Design review of the part built by this model. Coordinates are the model's own, in mm. A direction names the side the tool comes from. Give positions to 0.01 mm unless a question says otherwise; leave off trailing zeros. Write each loop counter-clockwise with the first axis right and the second up, starting at its lowest first coordinate (ties: lowest second). Pieces come first, ordered by that corner, then holes. Notation, with made-up numbers: M -25,84 L -8,84 A34 ccw -8,120 Z; hole C 68.25,17 d5. An arc over 180 degrees is marked long. Answer in a Markdown table with one row per item.
```python
from build123d import *

# Parameters (mm, degrees)
F1_DEPTH = 10
F2_R     = 5
F3_R     = 2.5
F5_R     = 1.5
F6_DEPTH = 25


# Not quite as in the source:
# - two fillets or chamfers of one size are made in one step
# - a feature names something its author has since deleted; it is built from what else it names


with BuildPart() as f1:
    # F0 (on Front) → F1 (new body)
    with BuildSketch(Plane.XZ):
        Polygon((-40.5, 0), (0, 0), (0, -6.2), (7, -6.2), (7, 7.8), (-47.5, 7.8), (-47.5, -6.2), (-87.5, -46.2), (-107.5, -46.2), (-107.5, -56.2), (-87.6005050634, -56.2), (-43.6005050634, -12.2), (-34.5, -12.2), (-34.5, -6.2), (-40.5, -6.2), align=None)
    extrude(amount=F1_DEPTH)

    # F2
    f2_edges = [f1.edges().sort_by_distance(p)[0] for p in [
        (7, -5, -6.2),
        (7, -5, 7.8),
        (-47.5, -5, 7.8),
        (-47.5, -5, -6.2),
        (-87.5, -5, -46.2),
        (-87.600505, -5, -56.2),
        (-43.600505, -5, -12.2),
    ]]
    fillet(f2_edges, radius=F2_R)

    # F3
    f3_edges = [f1.edges().sort_by_distance(p)[0] for p in [
        (-34.5, -5, -12.2),
        (-34.5, -5, -6.2),
    ]]
    fillet(f3_edges, radius=F3_R)

    # F5 (on face) → F6 (cut)
    with BuildSketch(Plane(origin=(0, 0, -56.2), x_dir=(1, 0, 0), z_dir=(0, 0, -1))):
        with Locations((-102.5, 5)):
            Circle(F5_R)
        with Locations((-92.5, 5)):
            Circle(F5_R)
    extrude(amount=-F6_DEPTH, mode=Mode.SUBTRACT)


solid = f1.part
```
1) To check wall thickness, follow probe 1 along Y at (x, z) = (-92.5, -52.5); probe 2 along X at (y, z) = (-0.75, -1); probe 3 along Z at (x, y) = (-1, -8.5). State the ranges of each line that lie inside material, in increasing order. Write a range as [from, to].
Geometry says:
| item | result |
|---|---|
| probe 1 | [-10, -6.5], [-3.5, 0] |
| probe 2 | [-47.5, -40.5], [0, 7] |
| probe 3 | [0, 7.8] |
2) The part is to be moulded in two halves that separate along Z. For faces 5 (the face through (7, -5, 1)), 6 (the face through (-39, -5, -6.2)), 7 (the face through (-35.252, -5.07, -6.913)), 8 (the face through (-87.63, -5.07, -45.81)), say which applies: released by +Z, released by -Z, zero draft, split by the parting line, or undercut.
Geometry says:
| item | result |
|---|---|
| face 5 | zero draft |
| face 6 | undercut |
| face 7 | undercut |
| face 8 | released by +Z |
3) Add section C-C (x = -29). Write out the cut boundary in (y, z), and give its area (3 significant figures).
Geometry says:
| item | result |
|---|---|
| outline | M -10,0 L 0,0 L 0,7.8 L -10,7.8 Z |
| area | 78.0 mm^2 |
4) Insertion check: P1, Ø1.6, axis at x = 1, y = -5, coming from the -Z side; P2, Ø1.9, axis at y = -4.5, z = -2.5, coming from the +X side; P3, Ø6, axis at y = -4, z = -26, coming from the -X side. Each pin has a flat end and moves straight along its axis. Give the tip position at first contact, or say it passes through.
Geometry says:
| item | result |
|---|---|
| P1 | z = -6.2 |
| P2 | x = 6.99 |
| P3 | x = -70.3 |
5) Add section B-B (y = -5). Count the separate pieces of the cut face and the enclosed holes in it, and give its area (3 significant figures).
Geometry says:
| item | result |
|---|---|
| separate pieces | 3 |
| enclosed holes | 0 |
| area | 1,120 mm^2 |
6) Add section A-A (x = -102.5). Write out the cut boundary in (y, z).
Geometry says:
| item | result |
|---|---|
| outline | M -10,-56.2 L -6.5,-56.2 L -6.5,-46.2 L -10,-46.2 Z; M -3.5,-56.2 L 0,-56.2 L 0,-46.2 L -3.5,-46.2 Z |
7) For faces 1 (the face through (-47.5, -5, -1)), 2 (the face through (-39, -5, -12.2)), 3 (the face through (0, -5, -3)), 4 (the face through (-107.5, -5, -51)), list the 3-axis set-ups (+Z, -Z, +X, -X, +Y, -Y) from which the entire face can be reached by the end or side of a thin tool; tool diameter is ignored.
Geometry says:
| item | result |
|---|---|
| face 1 | +Z, -X, +Y, -Y |
| face 2 | -Z, +X, +Y, -Y |
| face 3 | -Z, +Y, -Y |
| face 4 | +Z, -Z, -X, +Y, -Y |
8) Add section D-D (z = -33). Write out the cut boundary in (x, y), and give its area (3 significant figures).
Geometry says:
| item | result |
|---|---|
| outline | M -74.3,-10 L -64.4,-10 L -64.4,0 L -74.3,0 Z |
| area | 99.0 mm^2 |
